Geometry: final body of the model. Coordinates: model frame, mm. Face numbers are marked on the shaded views. Give positions to 0.01 mm unless a question says otherwise; leave off trailing zeros. Write each loop counter-clockwise with the first axis right and the second up, starting at its lowest first coordinate (ties: lowest second). Pieces come first, ordered by that corner, then holes. Notation, with made-up numbers: (-34, 78) -> (-1, 78) arc R10 cw to (-1, 93) -> close; hole circle Ø10 at (43, 67.25). An arc over 180 degrees is marked (long way). Answer in a Markdown table with one row per item. Add a question column.
Item 1: Draft query along Z for the marked faces 1, 2 and 3. Return one class per face: +Z half, -Z half, draft (parallel to the pull), parting line (faces both ways), or undercut.
Item 2: Section query B-B on x = -14.5. Output: boundary loops of the cut face in (y, z).
Item 3: Material intervals for probe 1 along Y at (x, z) = (-18.6, -10); probe 2 along X at (y, z) = (1.75, -10), sorted ascending. Write a range as from..to.
Item 4: Section query A-A on y = 14.5. Output: boundary loops of the cut face in (x, z), plus the area to 3 significant figures.
Item 5: Section query C-C on z = -3.25. Output: boundary loops of the cut face in (x, y), plus the area to 3 significant figures.
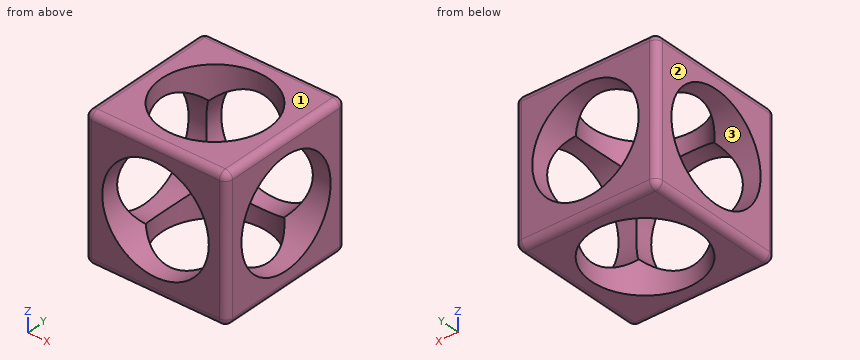
Autodesk Inventor part; units mm, degrees
ref_plane "YZ Plane" through (0, 0, 0) normal (1, 0, 0) x (0, 1, 0)
ref_plane "XZ Plane" through (0, 0, 0) normal (0, 1, 0) x (-1, 0, 0)
ref_plane "XY Plane" through (0, 0, 0) normal (0, 0, 1) x (1, 0, 0)
sketch "Эскиз1" plane through (0, 0, 0) normal (0, 1, 0) x (-1, 0, 0)
  line L0 (0, 0) -> (20, 0)
  line L1 (20, 0) -> (20, -20)
  line L2 (20, -20) -> (0, -20)
  line L3 (0, -20) -> (0, 0)
  dimension "d0" = 20
  dimension "d1" = 20
extrude "Выдавливание1" add sketch "Эскиз1" along normal blind 20
sketch "Эскиз2" plane through (0, 20, 0) normal (0, 1, 0) x (1, 0, 0)
  circle A0 centre (-10, 10) radius 7.5
  line L0 (0, 0) -> (0, 20)
  dimension "d4" = 15
  dimension "d5" = 10
  dimension "d6" = 10
sketch "Эскиз3" plane through (0, 0, -20) normal (0, 0, -1) x (-1, 0, 0)
  circle A0 centre (10, 10) radius 7.5
  line L0 (0, 0) -> (0, 20)
  line L1 (0, 0) -> (20, 0)
  dimension "d7" = 15
  dimension "d8" = 10
  dimension "d9" = 10
sketch "Эскиз4" plane through (0, 0, 0) normal (1, 0, 0) x (0, 0, -1)
  circle A0 centre (10, 10) radius 7.5
  line L0 (20, 0) -> (20, 20)
  line L1 (0, 20) -> (20, 20)
  point P0 (0, 0)
  dimension "d10" = 15
  dimension "d11" = 10
  dimension "d12" = 10
extrude "Выдавливание2" cut sketch "Эскиз2" against normal blind 20
extrude "Выдавливание3" cut sketch "Эскиз4" against normal blind 20
extrude "Выдавливание4" cut sketch "Эскиз3" against normal blind 20
fillet "Сопряжение1" radius 1 12 edges at (0, 0, -10) (-10, 0, -20) (0, 10, -20) (0, 20, -10) (-10, 20, -20) (-20, 20, -10) (-20, 0, -10) (-10, 0, 0) (-10, 20, 0) (0, 10, 0) (-20, 10, 0) (-20, 10, -20)
properties part number "КубСоединительный2020"
Findings below:
| question | item | result |
|---|---|---|
| 1 | face 1 | +Z half |
| 1 | face 2 | draft |
| 1 | face 3 | undercut |
| 2 | outline | (0, -19) arc R1 ccw to (1, -20) -> (4, -20) -> (4, -16) -> (0, -16) -> close; (0, -4) -> (4, -4) -> (4, 0) -> (1, 0) arc R1 ccw to (0, -1) -> close; (16, -20) -> (19, -20) arc R1 ccw to (20, -19) -> (20, -16) -> (16, -16) -> close; (16, -4) -> (20, -4) -> (20, -1) arc R1 ccw to (19, 0) -> (16, 0) -> close |
| 3 | probe 1 | y = 0..2.5, 17.5..20 |
| 3 | probe 2 | x = -20..-17.5, -2.5..0 |
| 4 | outline | (-20, -19) arc R1 ccw to (-19, -20) -> (-16, -20) -> (-16, -16) -> (-20, -16) -> close; (-20, -4) -> (-16, -4) -> (-16, 0) -> (-19, 0) arc R1 ccw to (-20, -1) -> close; (-4, -20) -> (-1, -20) arc R1 ccw to (0, -19) -> (0, -16) -> (-4, -16) -> close; (-4, -4) -> (0, -4) -> (0, -1) arc R1 ccw to (-1, 0) -> (-4, 0) -> close |
| 4 | area | 63.1 mm^2 |
| 5 | outline | (-20, 1) arc R1 ccw to (-19, 0) -> (-13.27, 0) -> (-13.27, 3.25) arc R7.5 cw to (-16.75, 6.73) -> (-20, 6.73) -> close; (-20, 13.27) -> (-16.75, 13.27) arc R7.5 cw to (-13.27, 16.75) -> (-13.27, 20) -> (-19, 20) arc R1 ccw to (-20, 19) -> close; (-6.73, 0) -> (-1, 0) arc R1 ccw to (0, 1) -> (0, 6.73) -> (-3.25, 6.73) arc R7.5 cw to (-6.73, 3.25) -> close; (-6.73, 16.75) arc R7.5 cw to (-3.25, 13.27) -> (0, 13.27) -> (0, 19) arc R1 ccw to (-1, 20) -> (-6.73, 20) -> close |
| 5 | area | 151 mm^2 |
